CAD build for the part. Positions are in the model's coordinates, mm. A direction names the side the tool comes from. Round coordinates to 2 decimals unless told otherwise and drop trailing zeros. Loops run counter-clockwise (first coordinate to the right, second up) from the corner with the lowest first, then second, coordinate; pieces in that order, holes last. Notation, with made-up numbers: (-35.5, 5) - (20.5, 5) arc R25 cw to (20.5, 41) - close; hole circle Ø9 at (64.25, -25). An arc over 180 degrees is marked (long way). Use one line per item in the form item = value.
from build123d import *

# Parameters (mm, degrees)
SKETCH1_W           = 15
SKETCH1_H           = 60
BOSS_EXTRUDE1_DEPTH = 70
SKETCH2_R           = 17
CUT_EXTRUDE1_DEPTH  = 70
SKETCH3_W           = 60
SKETCH3_H           = 40
CUT_EXTRUDE2_DEPTH  = 29
SKETCH4_R           = 1.5
CUT_EXTRUDE3_DEPTH  = 43
SKETCH5_R           = 2
CUT_EXTRUDE4_DEPTH  = 10
SKETCH7_R           = 3
CUT_EXTRUDE5_DEPTH  = 10
FILLET1_R           = 5


with BuildPart() as part:
    # Sketch1 → Boss-Extrude1 (new body)
    with BuildSketch(Plane(origin=(0, 0, 0), x_dir=(1, 0, 0), z_dir=(0, 1, 0))):
        Rectangle(SKETCH1_W, SKETCH1_H)
    extrude(amount=BOSS_EXTRUDE1_DEPTH)

    # Sketch2 → Cut-Extrude1 (cut)
    with BuildSketch(Plane(origin=(7.5, 0, 0), x_dir=(0, 0, -1), z_dir=(1, 0, 0))):
        with Locations((0, 30)):
            Circle(SKETCH2_R)
    extrude(amount=-CUT_EXTRUDE1_DEPTH, mode=Mode.SUBTRACT)

    # Sketch3 → Cut-Extrude2 (cut)
    with BuildSketch(Plane(origin=(7.5, 0, 0), x_dir=(0, 0, -1), z_dir=(1, 0, 0))):
        with Locations((0, 50)):
            Rectangle(SKETCH3_W, SKETCH3_H)
    extrude(amount=-CUT_EXTRUDE2_DEPTH, mode=Mode.SUBTRACT)

    # Sketch4 → Cut-Extrude3 (cut)
    with BuildSketch(Plane(origin=(0, 30, 0), x_dir=(1, 0, 0), z_dir=(0, 1, 0))):
        with Locations(Location((-4, 24, 0), (0, 0, 270))):
            Circle(SKETCH4_R)
        with Locations(Location((4, 24, 0), (0, 0, 270))):
            Circle(SKETCH4_R)
        with Locations(Location((-4, -24, 0), (0, 0, 270))):
            Circle(SKETCH4_R)
        with Locations(Location((4, -24, 0), (0, 0, 270))):
            Circle(SKETCH4_R)
    extrude(amount=-CUT_EXTRUDE3_DEPTH, mode=Mode.SUBTRACT)

    # Sketch5 → Cut-Extrude4 (cut)
    with BuildSketch(Plane(origin=(7.5, 0, 0), x_dir=(0, 0, -1), z_dir=(1, 0, 0))):
        with Locations((-16, 14)):
            Circle(SKETCH5_R)
        with Locations((16, 14)):
            Circle(SKETCH5_R)
    extrude(amount=-CUT_EXTRUDE4_DEPTH, mode=Mode.SUBTRACT)

    # Sketch7 → Cut-Extrude5 (cut)
    with BuildSketch(Plane.XZ):
        with Locations(Location((-4, 24, 0), (0, 0, 270))):
            Circle(SKETCH7_R)
        with Locations(Location((4, 24, 0), (0, 0, 270))):
            Circle(SKETCH7_R)
        with Locations(Location((-4, -24, 0), (0, 0, 270))):
            Circle(SKETCH7_R)
        with Locations(Location((4, -24, 0), (0, 0, 270))):
            Circle(SKETCH7_R)
    extrude(amount=-CUT_EXTRUDE5_DEPTH, mode=Mode.SUBTRACT)

    # Fillet1
    # the kernel refuses this fillet: 5 mm, written as the material it takes off along each edge
    with BuildSketch(Plane(origin=(-20, 0, -30), x_dir=(0, 0, 1), z_dir=(1, 0, 0))) as fillet1_piece_1:
        with BuildLine():
            CenterArc((FILLET1_R, -FILLET1_R), FILLET1_R, 90, 90)
            Line((0, -FILLET1_R), (0, 0))
            Line((0, 0), (FILLET1_R, 0))
        make_face()
    extrude(amount=40, mode=Mode.SUBTRACT)
    with BuildSketch(Plane(origin=(20, 0, 30), x_dir=(0, 1, 0), z_dir=(-1, 0, 0))) as fillet1_piece_2:
        with BuildLine():
            CenterArc((FILLET1_R, FILLET1_R), FILLET1_R, 180, 90)
            Line((0, FILLET1_R), (0, 0))
            Line((0, 0), (FILLET1_R, 0))
        make_face()
    extrude(amount=40, mode=Mode.SUBTRACT)


solid = part.part
1) Slice it at C-C (z = 0). Write the cut outline in (x, y), plus the area to 3 significant figures.
Report:
outline = (-7.5, 0) - (7.5, 0) - (7.5, 13) - (-7.5, 13) - close
area = 195 mm^2
2) Two-plate mould, pull along Z, no slides. Class faces 1 (the flat face through (0, 30, 24)), 2 (the cylindrical face through (0, 2, -29)), 3 (the cylindrical face through (2.57, 15.352, -14.526)), 4 (the cylindrical face through (-4, 5, 27)): +Z half, -Z half, draft (parallel to the pull), parting line (faces both ways), or undercut.
Report:
face_1 = draft
face_2 = -Z half
face_3 = undercut
face_4 = undercut
3) Slice it at B-B (y = 6). Write the cut outline in (x, z), plus the area to 3 significant figures.
Report:
outline = (-7.5, -30) - (7.5, -30) - (7.5, 30) - (-7.5, 30) - close; hole circle Ø6 at (-4, -24); hole circle Ø6 at (-4, 24); hole circle Ø6 at (4, -24); hole circle Ø6 at (4, 24)
area = 787 mm^2
4) Tool access for faces 5 (the cylindrical face through (-3.93, 20.14, -25.5)), 6 (the flat face through (2.7, 10, 22.7)), 7 (the flat face through (-2.5, 14, -16)): list every direction of +Z, -Z, +X, -X, +Y, -Y with a clear straight run to the whole face (end or side of a thin tool).
Report:
face_5 = +Y, -Y
face_6 = -Y
face_7 = +X
5) Slice it at D-D (z = -15.5). Write the cut outline in (x, y), plus the area to 3 significant figures.
Report:
outline = (-7.5, 0) - (7.5, 0) - (7.5, 12.06) - (-2.5, 12.06) - (-2.5, 15.94) - (7.5, 15.94) - (7.5, 23.02) - (-7.5, 23.02) - close
area = 307 mm^2
6) Drill centre lines: probe 1 along X at (y, z) = (17, -24); probe 2 along Z at (x, y) = (-4.25, 6.5); probe 3 along X at (y, z) = (2, -24). Where is each one in solid material? Low to high.
Report:
probe_1 = -7.5 to -5.5, -2.5 to 2.5, 5.5 to 7.5
probe_2 = -30 to -26.99, -21.01 to 21.01, 26.99 to 30
probe_3 = -7.5 to -7, -1 to 1, 7 to 7.5
7) Slice it at A-A (z = 24). Write the cut outline in (x, y).
Report:
outline = (-7.5, 0) - (-7, 0) - (-7, 10) - (-5.5, 10) - (-5.5, 30) - (-7.5, 30) - close; (-2.5, 10) - (-1, 10) - (-1, 0) - (1, 0) - (1, 10) - (2.5, 10) - (2.5, 30) - (-2.5, 30) - close; (5.5, 10) - (7, 10) - (7, 0) - (7.5, 0) - (7.5, 30) - (5.5, 30) - close
8) Flat gauge pins, fed straight in: pin 1 (6 mm diameter, centred on x = 5, z = -11.5, fed in from +Y); pin 2 (3.5 mm diameter, centred on x = -4, z = -24, fed in from -Y); pin 3 (1 mm diameter, centred on x = -6, z = -11.5, fed in from +Y); pin 4 (5 mm diameter, centred on x = -4.5, z = -23.5, fed in from -Y). Where does each tip first touch, or does it go through?
Report:
pin_1 = 21.13
pin_2 = 10
pin_3 = 17.96
pin_4 = 0
